Part model, mm, in its own coordinate system. A direction names the side the tool comes from. Round coordinates to 2 decimals unless told otherwise and drop trailing zeros. Write each loop counter-clockwise with the first axis right and the second up, starting at its lowest first coordinate (ties: lowest second). Pieces come first, ordered by that corner, then holes.
1) Which spindle directions (+Z, -Z, +X, -X, +Y, -Y) get a long thin tool onto all of the face, cutting with end or side? Do faces 4 (the cylindrical face through (35.277, -4.782, 27.059)), 5 (the cylindrical face through (-73.02, -12.74, 22.31)). Say none if no direction does.
2) Flat gauge pins, fed straight in: pin 1 (5 mm diameter, centred on x = 21, z = -40.65, fed in from +Y); pin 2 (6.5 mm diameter, centred on x = 33.25, z = 25.2, fed in from -Y). Where does each tip first touch, or does it go through?
3) Saw through at C-C on x = -33.25. Count the separate pieces of the cut face and the enclosed holes in it, and give its area (3 significant figures).
4) Drill centre lines: L1, parallel to X at y = -10.5, z = -120; L2, parallel to Z at x = -33.25, y = -11; L3, parallel to Z at x = -69.25, y = -3.25. Where is each one in solid material? Low to high.
5) Saw through at B-B on x = -3. Write the cut outline in (y, z), and give its area (3 significant figures).
6) Pull direction X, two halves, no side cores. Call faces 1 (the cylindrical face through (-34.28, -12.742, -151.137)), 2 (the flat face through (-1, -15.7, 2)), 3 (the flat face through (-1, -6.7, -43)): +X half, -X half, draft (parallel to the pull), parting line (faces both ways), or undercut.
7) Saw through at A-A on z = -40.65. Write the cut outline in (x, y), and give its area (3 significant figures).
```python
from build123d import *

# Parameters (mm, degrees)
SKETCH_W             = 152.5
SKETCH_H             = 305
PAD_DEPTH            = 15.7
SKETCH001_R          = 2.1
POCKET_DEPTH         = 682.724194
POCKET_DEPTH_BACK    = 698.424194
SKETCH002_R          = 2.4
POCKET001_DEPTH      = 0.001
POCKET001_DEPTH_BACK = 15.701
HOLE003_D            = 5.5
HOLE003_CBORE_D      = 9.5
HOLE003_CBORE_DEPTH  = 6
SKETCH011_R          = 2.1
POCKET002_DEPTH      = 15
HOLE004_D            = 5.5
HOLE004_CBORE_D      = 9.5
HOLE004_CBORE_DEPTH  = 9
SKETCH014_R          = 2.5
POCKET004_DEPTH      = 30


with BuildPart() as part:
    # Sketch → Pad (new body)
    with BuildSketch(Plane.XZ):
        Rectangle(SKETCH_W, SKETCH_H)
    extrude(amount=PAD_DEPTH)

    # Sketch001 → Pocket (cut, two sides)
    with BuildSketch(Plane.XZ) as pocket_sk:
        with Locations((-54, 0)):
            Circle(SKETCH001_R)
        with Locations((-54, 60)):
            Circle(SKETCH001_R)
        with Locations((-54, 120)):
            Circle(SKETCH001_R)
        with Locations((-54, -60)):
            Circle(SKETCH001_R)
        with Locations((-54, -120)):
            Circle(SKETCH001_R)
    pocket = extrude(amount=-POCKET_DEPTH, mode=Mode.SUBTRACT) + extrude(pocket_sk.sketch, amount=POCKET_DEPTH_BACK, mode=Mode.SUBTRACT)

    # Mirrored: Pocket across Sketch001 V_Axis
    add(pocket.mirror(Plane(origin=(0, 0, 0), x_dir=(0, -1, 0), z_dir=(1, 0, 0))), mode=Mode.SUBTRACT)

    # Sketch002 → Pocket001 (cut, two sides)
    with BuildSketch(Plane.XZ) as pocket001_sk:
        with Locations((-23, -120.525)):
            Circle(SKETCH002_R)
        with Locations((23, -120.525)):
            Circle(SKETCH002_R)
        with Locations((-23, 88.475)):
            Circle(SKETCH002_R)
        with Locations((-23, 75.475)):
            Circle(SKETCH002_R)
        with Locations((23, 88.475)):
            Circle(SKETCH002_R)
        with Locations((23, 75.475)):
            Circle(SKETCH002_R)
    extrude(amount=-POCKET001_DEPTH, mode=Mode.SUBTRACT)
    extrude(pocket001_sk.sketch, amount=POCKET001_DEPTH_BACK, mode=Mode.SUBTRACT)

    # Hole003 (through all)
    with Locations(Plane.XZ.offset(15.7)):
        with Locations((-69.25, -146.5), (-69.25, -114.5), (-33.25, -114.5), (-33.25, -146.5), (33.25, -114.5), (69.25, -114.5), (33.25, -146.5), (69.25, -146.5), (-69.25, -6.8), (-69.25, 25.2), (-33.25, -6.8), (-33.25, 25.2), (33.25, -6.8), (33.25, 25.2), (69.25, -6.8), (69.25, 25.2)):
            CounterBoreHole(HOLE003_D / 2, HOLE003_CBORE_D / 2, HOLE003_CBORE_DEPTH)

    # Sketch011 (on Face1 of Hole003) → Pocket002 (cut)
    with BuildSketch(Plane(origin=(0, 0, 152.5), x_dir=(-1, 0, 0), z_dir=(0, 0, 1))):
        with Locations((-60, 7.85)):
            Circle(SKETCH011_R)
        with Locations((-20, 7.85)):
            Circle(SKETCH011_R)
        with Locations((20, 7.85)):
            Circle(SKETCH011_R)
        with Locations((60, 7.85)):
            Circle(SKETCH011_R)
    extrude(amount=-POCKET002_DEPTH, mode=Mode.SUBTRACT)

    # Hole004 (through all)
    with Locations(Plane.XZ.offset(15.7)):
        with Locations((-3, -40.65), (21, -40.65), (-3, -80.65), (21, -80.65)):
            CounterBoreHole(HOLE004_D / 2, HOLE004_CBORE_D / 2, HOLE004_CBORE_DEPTH)

    # Sketch014 (on Face2 of Hole004) → Pocket004 (cut)
    with BuildSketch(Plane(origin=(-76.25, 0, 0), x_dir=(0, 0, -1), z_dir=(-1, 0, 0))):
        with Locations((26.5, 7.85)):
            Circle(SKETCH014_R)
    extrude(amount=-POCKET004_DEPTH, mode=Mode.SUBTRACT)


solid = part.part
```
Completed:
1. face 4: +Y, -Y
1. face 5: -Y
2. pin 1: passes through
2. pin 2: stops at y = -9.7
3. separate pieces: 5
3. enclosed holes: 0
3. area: 4,350 mm2
4. L1: x = -76.25 to -56.1, -51.9 to -25.34, -20.66 to 20.66, 25.34 to 51.9, 56.1 to 76.25
4. L2: z = -152.5 to -151.25, -141.75 to -119.25, -109.75 to -11.55, -2.05 to 20.45, 29.95 to 152.5
4. L3: z = -152.5 to -149.25, -143.75 to -117.25, -111.75 to -9.55, -4.05 to 22.45, 27.95 to 152.5
5. outline: (-15.7, -152.5) - (0, -152.5) - (0, -83.4) - (-6.7, -83.4) - (-6.7, -85.4) - (-15.7, -85.4) - close; (-15.7, -75.9) - (-6.7, -75.9) - (-6.7, -77.9) - (0, -77.9) - (0, -43.4) - (-6.7, -43.4) - (-6.7, -45.4) - (-15.7, -45.4) - close; (-15.7, -35.9) - (-6.7, -35.9) - (-6.7, -37.9) - (0, -37.9) - (0, 152.5) - (-15.7, 152.5) - close
5. area: 4,540 mm2
6. face 1: undercut
6. face 2: draft
6. face 3: undercut
7. outline: (-76.25, -15.7) - (-7.75, -15.7) - (-7.75, -6.7) - (-5.75, -6.7) - (-5.75, 0) - (-76.25, 0) - close; (-0.25, -6.7) - (1.75, -6.7) - (1.75, -15.7) - (16.25, -15.7) - (16.25, -6.7) - (18.25, -6.7) - (18.25, 0) - (-0.25, 0) - close; (23.75, -6.7) - (25.75, -6.7) - (25.75, -15.7) - (76.25, -15.7) - (76.25, 0) - (23.75, 0) - close
7. area: 2,150 mm2
